Geometry check sheet. Reference: the model listing, model coordinates, mm. Face numbers are marked on the shaded views. A direction names the side the tool comes from. Coordinates: 2 decimals unless noted, no trailing zeros. Write each loop counter-clockwise with the first axis right and the second up, starting at its lowest first coordinate (ties: lowest second). Pieces come first, ordered by that corner, then holes.
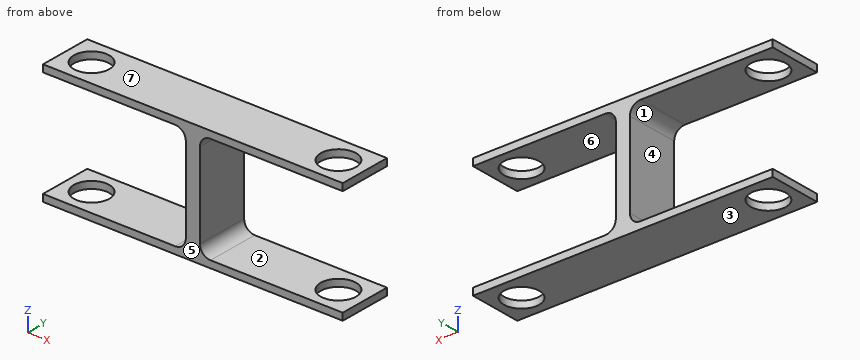
from build123d import *

# Parameters (mm, degrees)
SKETCH1_W           = 215.9
SKETCH1_H           = 38.1
BOSS_EXTRUDE1_DEPTH = 5.08
SKETCH2_R           = 12.7
CUT_EXTRUDE1_DEPTH  = 110.735643252
SKETCH3_W           = 10.16
SKETCH3_H           = 38.1
BOSS_EXTRUDE2_DEPTH = 38.1
FILLET1_R           = 7.62


with BuildPart() as part:
    # Sketch1 → Boss-Extrude1 (new body)
    with BuildSketch(Plane.XY):
        Rectangle(SKETCH1_W, SKETCH1_H)
    boss_extrude1 = extrude(amount=BOSS_EXTRUDE1_DEPTH)

    # Sketch2 → Cut-Extrude1 (cut, through all)
    with BuildSketch(Plane.XY):
        with Locations((-88.9, 0)):
            Circle(SKETCH2_R)
        with Locations((88.9, 0)):
            Circle(SKETCH2_R)
    cut_extrude1 = extrude(amount=CUT_EXTRUDE1_DEPTH, mode=Mode.SUBTRACT)

    # Sketch3 → Boss-Extrude2 (add)
    with BuildSketch(Plane.XY):
        Rectangle(SKETCH3_W, SKETCH3_H)
    boss_extrude2 = extrude(amount=-BOSS_EXTRUDE2_DEPTH)

    # Mirror2: Boss-Extrude2 across plane
    add(boss_extrude2.mirror(Plane(origin=(0, 0, -38.1), x_dir=(1, 0, 0), z_dir=(0, 0, -1))))

    # Mirror3: Boss-Extrude1, Cut-Extrude1 across plane
    add(boss_extrude1.mirror(Plane(origin=(0, 0, -38.1), x_dir=(1, 0, 0), z_dir=(0, 0, -1))))
    add(cut_extrude1.mirror(Plane(origin=(0, 0, -38.1), x_dir=(1, 0, 0), z_dir=(0, 0, -1))), mode=Mode.SUBTRACT)

    # Fillet1
    fillet1_edges = [part.edges().sort_by_distance(p)[0] for p in [
        (5.08, 0, 0),
        (-5.08, 0, 0),
        (5.08, 0, -76.2),
        (-5.08, 0, -76.2),
    ]]
    fillet(fillet1_edges, radius=FILLET1_R)


solid = part.part
1. Gauge pin test, flat ends, axial feed: pin 1 Ø2 at (y, z) = (7.5, -5.5) entering from +X; pin 2 Ø1 at (y, z) = (-9, -6) entering from -X; pin 3 Ø2 at (y, z) = (-1, -43.5) entering from +X. Record the tip position at first contact, or that the pin passes through.
Computed values:
pin 1: stops at x = 5.75
pin 2: stops at x = -5.38
pin 3: stops at x = 5.08
2. Sectioned sample at C-C, the plane x = -88.9. Record the boundary of the cut face in (y, z).
Computed values:
outline: (-19.05, -81.28) - (-12.7, -81.28) - (-12.7, -76.2) - (-19.05, -76.2) - close; (-19.05, 0) - (-12.7, 0) - (-12.7, 5.08) - (-19.05, 5.08) - close; (12.7, -81.28) - (19.05, -81.28) - (19.05, -76.2) - (12.7, -76.2) - close; (12.7, 0) - (19.05, 0) - (19.05, 5.08) - (12.7, 5.08) - close
3. Sectioned sample at B-B, the plane x = -18.5. Record the boundary of the cut face in (y, z).
Computed values:
outline: (-19.05, -81.28) - (19.05, -81.28) - (19.05, -76.2) - (-19.05, -76.2) - close; (-19.05, 0) - (19.05, 0) - (19.05, 5.08) - (-19.05, 5.08) - close
4. Draft check along Z on the marked faces 4, 5, 6 and 7. Enter one of: released by +Z, released by -Z, zero draft, split by the parting line, or undercut.
Computed values:
face 4: undercut
face 5: zero draft
face 6: undercut
face 7: released by +Z
5. Sectioned sample at A-A, the plane y = 0. Give the number of separate pieces and of enclosed holes in the cut face, and give its area (3 significant figures).
Computed values:
separate pieces: 5
enclosed holes: 0
area: 2,500 mm2
6. Access from +Z, -Z, +X, -X, +Y, -Y to the whole of each face (thin tool, end or side, straight path). Record for the marked faces 1, 2 and 3.
Computed values:
face 1: -X, +Y, -Y
face 2: +X, +Y, -Y
face 3: -Z, +X, -X, +Y, -Y
7. Thickness scan on line 1 along X through (y, z) = (0, 1); line 2 along Z through (x, y) = (48.5, 14); line 3 along Y through (x, z) = (88.9, 1.15). Record the ranges inside material, lowest first.
Computed values:
line 1: x = -107.95 to -101.6, -76.2 to 76.2, 101.6 to 107.95
line 2: z = -81.28 to -76.2, 0 to 5.08
line 3: y = -19.05 to -12.7, 12.7 to 19.05
